```python
from build123d import *

# Parameters (mm, degrees)
SKETCH_W        = 7.5
SKETCH_H        = 6.9
PAD_DEPTH       = 5.75
THICKNESS_T     = -0.7
POCKET_DEPTH    = 0.7
POCKET001_DEPTH = 7.501
PAD004_DEPTH    = 6.1
SKETCH005_W     = 1.7
SKETCH005_H     = 0.6
POCKET002_DEPTH = 7.001
PAD005_DEPTH    = 5.9


with BuildPart() as part:
    # Sketch → Pad (new body)
    with BuildSketch(Plane.XY):
        Rectangle(SKETCH_W, SKETCH_H)
    extrude(amount=PAD_DEPTH)

    # Thickness
    thickness_openings = [part.faces().sort_by_distance(p)[0] for p in [
        (0, -3.45, 2.875),
    ]]
    offset(amount=THICKNESS_T, openings=thickness_openings, kind=Kind.INTERSECTION)

    # Sketch001 (on Face5 of Thickness) → Pocket (cut)
    with BuildSketch(Plane.XY.offset(5.75)):
        with BuildLine():
            Line((1.75, -2.75), (1.75, 0.1))
            ThreePointArc((1.75, 0.1), (1.647487, 0.347487), (1.4, 0.45))
            Line((1.4, 0.45), (-1.4, 0.45))
            ThreePointArc((-1.4, 0.45), (-1.647487, 0.347487), (-1.75, 0.1))
            Line((-1.75, 0.1), (-1.75, -2.75))
            ThreePointArc((-1.75, -2.75), (-1.647487, -2.997487), (-1.4, -3.1))
            Line((-1.4, -3.1), (-1.75, -3.45))
            Line((-1.75, -3.45), (1.75, -3.45))
            Line((1.4, -3.1), (1.75, -3.45))
            ThreePointArc((1.4, -3.1), (1.647487, -2.997487), (1.75, -2.75))
        make_face()
    extrude(amount=-POCKET_DEPTH, mode=Mode.SUBTRACT)

    # Sketch002 (on Face2 of Pocket) → Pocket001 (cut, through all)
    with BuildSketch(Plane(origin=(-3.75, 0, 0), x_dir=(0, -1, 0), z_dir=(-1, 0, 0))):
        with BuildLine():
            Line((0.95, 5.05), (3.45, 5.05))
            Line((3.45, 5.05), (3.45, 4.05))
            Line((3.45, 4.05), (0.45, 4.05))
            Line((0.45, 4.55), (0.45, 4.05))
            ThreePointArc((0.95, 5.05), (0.596447, 4.903553), (0.45, 4.55))
        make_face()
    extrude(amount=-POCKET001_DEPTH, mode=Mode.SUBTRACT)

    # Sketch008 → Pad004 (join)
    with BuildSketch(Plane(origin=(3.05, 0, 0), x_dir=(0, -1, 0), z_dir=(-1, 0, 0))):
        Polygon((-2.75, 5.05), (-2.45, 5.05), (-2.45, 2.473205), (-2.75, 2.3), align=None)
    extrude(amount=PAD004_DEPTH)

    # Sketch005 → Pocket002 (cut, through all)
    with BuildSketch(Plane.XY.offset(7)):
        with Locations((-1.3, 3.15)):
            Rectangle(SKETCH005_W, SKETCH005_H)
        with Locations((1.3, 3.15)):
            Rectangle(SKETCH005_W, SKETCH005_H)
    extrude(amount=-POCKET002_DEPTH, mode=Mode.SUBTRACT)

    # Sketch009 (on ShapeBinder) → Pad005 (join)
    with BuildSketch(Plane(origin=(2.15, 0, 0), x_dir=(0, -1, 0), z_dir=(-1, 0, 0))):
        Polygon((-2.85, 5.75), (-3.45, 4.4), (-3.45, 2.5), (-2.85, 0), align=None)
    extrude(amount=PAD005_DEPTH)


solid = part.part
```
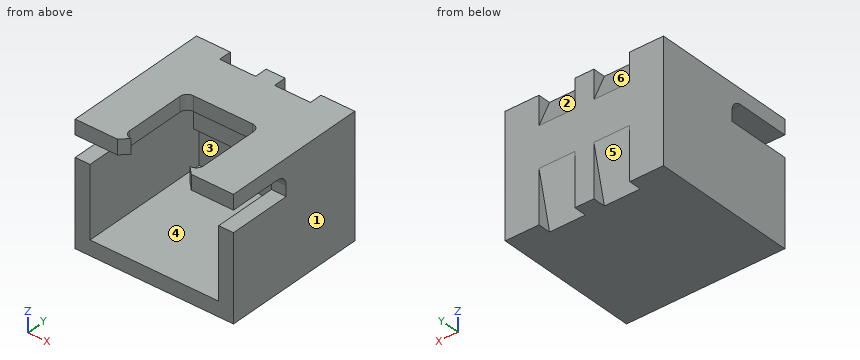
Build history of the part. All positions in model axes, mm. Face numbers are marked on the shaded views. A direction names the side the tool comes from. Give positions to 0.01 mm unless a question says otherwise; leave off trailing zeros. Order: outer loops, then holes, each group sorted by start corner. A loop starts at its lowest first (then second) coordinate and runs counter-clockwise, first axis right, second up. Notation, with made-up numbers: M -17,46.25 L 28,46.25 A17 ccw 28,60.25 Z; hole C 88.5,35.5 d6. An arc over 180 degrees is marked long. Return JSON: item names as keys, results as strings.
Q1. Band-saw the part on D-D (z = 4.15). Give the cut face in (x, y), then the cut area to 3 significant figures.
Answer list:
{"outline": "M -3.75,-0.45 L -3.05,-0.45 L -3.05,2.45 L 3.05,2.45 L 3.05,-0.45 L 3.75,-0.45 L 3.75,3.45 L -3.75,3.45 Z", "area": "11.6 mm^2"}
Q2. Wall check: probe 1 along X at (y, z) = (0.25, 1.95); probe 2 along Z at (x, y) = (-3.25, -1); probe 3 along Z at (x, y) = (-2.25, -2). Give the ranges that are in metal, low to high. Write a range as from..to.
Answer list:
{"probe 1": "x = -3.75..-3.05, 3.05..3.75", "probe 2": "z = 0..4.05, 5.05..5.75", "probe 3": "z = 0..0.7, 5.05..5.75"}
Q3. Band-saw the part on A-A (y = -2). Give the cut face in (x, z).
Answer list:
{"outline": "M -3.75,0 L 3.75,0 L 3.75,4.05 L 3.05,4.05 L 3.05,0.7 L -3.05,0.7 L -3.05,4.05 L -3.75,4.05 Z; M -3.75,5.05 L -1.75,5.05 L -1.75,5.75 L -3.75,5.75 Z; M 1.75,5.05 L 3.75,5.05 L 3.75,5.75 L 1.75,5.75 Z"}
Q4. Two-plate mould, pull along Z, no slides. Class the marked faces 1, 2 and 3: pulls with the +Z half, pulls with the -Z half, needs draft (parallel to the pull), parting line crosses it, or undercut.
Answer list:
{"face 1": "needs draft", "face 2": "pulls with the +Z half", "face 3": "undercut"}
Q5. Band-saw the part on B-B (x = -2.25). Give the cut face in (y, z), then the cut area to 3 significant figures.
Answer list:
{"outline": "M -3.45,0 L 3.45,0 L 3.45,5.75 L -3.45,5.75 L -3.45,5.05 L 2.45,5.05 L 2.45,2.47 L 2.75,2.3 L 2.75,0.7 L -3.45,0.7 Z", "area": "13.5 mm^2"}
Q6. Band-saw the part on C-C (y = 2). Give the cut face in (x, z), then the cut area to 3 significant figures.
Answer list:
{"outline": "M -3.75,0 L 3.75,0 L 3.75,5.75 L -3.75,5.75 Z; hole M -3.05,0.7 L 3.05,0.7 L 3.05,5.05 L -3.05,5.05 Z", "area": "16.6 mm^2"}
Q7. Flat gauge pin, fed straight in: pin 1 (0.5 mm diameter, centred on x = -1, z = 1, fed in from -Y). Where does the tip first touch, or does it go through?
Answer list:
{"pin 1": "stops at y = 2.75"}
Q8. 3-axis set-ups, long thin cutter, end or side, ignore diameter. For the marked faces 4, 5 and 6: which of +Z, -Z, +X, -X, +Y, -Y reach the whole face in a straight line?
Answer list:
{"face 4": "-Y", "face 5": "-Z, +Y", "face 6": "+Z, +Y"}
